The listing builds one solid part. Answer for the finished solid, in the listing's coordinates (mm). Face numbers are marked on the shaded views. A direction names the side the tool comes from. Round coordinates to 2 decimals unless told otherwise and drop trailing zeros. Write each loop counter-clockwise with the first axis right and the second up, starting at its lowest first coordinate (ties: lowest second). Pieces come first, ordered by that corner, then holes. Notation, with made-up numbers: M 15.5,19.25 L 56.5,19.25 A13 cw 56.5,40.25 Z; hole C -23.75,88.5 d3. An arc over 180 degrees is marked long. One line per item, written item: value. Start each with the question number.
(1) Section A-A (y = -11) is taken. Determine the outline of the cut face in (x, z), plus the area to 3 significant figures.
(2) Section C-C (y = -22) is taken. Determine the outline of the cut face in (x, z).
(3) Given P1, Ø0.7, axis at y = -26.5, z = 5, coming from the +X side; P2, Ø1.3, axis at x = 0, y = -22, coming from the -Z side; P3, Ø1, axis at y = -28, z = 4, coming from the +X side, each flat-ended and moving along its own axis, determine where each tip first touches the part or whether it passes through.
(4) For a pull along Y with two mould halves and no side action, classify the marked faces 1, 2, 3 and 4 as released by +Y, released by -Y, zero draft, split by the parting line, or undercut.
(5) For the marked faces 5, 6, 7 and 8, determine the directions among +Z, -Z, +X, -X, +Y, -Y from which every point of the face is accessible in a straight line to the end or side of a thin tool.
(6) Section B-B (x = 5) is taken. Determine the outline of the cut face in (y, z).
(7) Consider probe 1 along X at (y, z) = (-11, 1.55); probe 2 along X at (y, z) = (-12.5, 3); probe 3 along Y at (x, z) = (5, 2.8). Determine where each line is inside the solid, lowest interval first.
(8) Section D-D (z = 0.7) is taken. State how many separate pieces and enclosed holes the cut face has, plus the area to 3 significant figures.
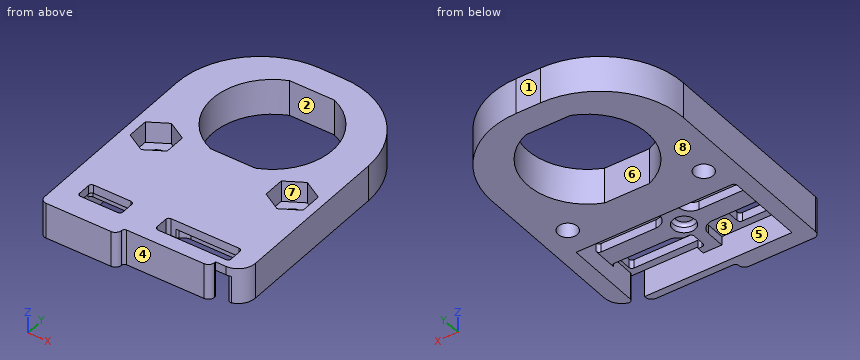
```python
from build123d import *

# Parameters (mm, degrees)
SKETCH_R        = 1.55
SKETCH_W        = 7
SKETCH_H        = 3
SKETCH_W_2      = 12
PAD_DEPTH       = 5.8
SKETCH005_W     = 25.7
SKETCH005_H     = 13
POCKET_DEPTH    = 3
SKETCH006_R     = 1.8
POCKET001_DEPTH = 1.4
POCKET002_DEPTH = 3.4
FILLET_R        = 1
FILLET001_R     = 0.5


with BuildPart() as part:
    # Sketch → Pad (new body)
    with BuildSketch(Plane.XY):
        with BuildLine():
            Line((-2, 13.5), (2, 13.5))
            ThreePointArc((15.5, 0), (11.545942, 9.545942), (2, 13.5))
            Line((15.5, 0), (15.5, -25.7))
            ThreePointArc((12.7, -28.5), (14.679899, -27.679899), (15.5, -25.7))
            Line((11, -28.5), (12.7, -28.5))
            Line((11, -29.7), (11, -28.5))
            Line((-3, -29.7), (11, -29.7))
            Line((-3, -31.15), (-3, -29.7))
            Line((-3, -31.15), (-15.5, -31.15))
            Line((-15.5, -31.15), (-15.5, 0))
            ThreePointArc((-2, 13.5), (-11.545942, 9.545942), (-15.5, 0))
        make_face()
        with Locations((-11, -11)):
            Circle(SKETCH_R, mode=Mode.SUBTRACT)
        with Locations((11, -11)):
            Circle(SKETCH_R, mode=Mode.SUBTRACT)
        with BuildLine():
            ThreePointArc((-3.618011, 9), (-9.7, 0), (-3.618011, -9))
            Line((3.618011, -9), (-3.618011, -9))
            ThreePointArc((3.618011, -9), (9.7, 0), (3.618011, 9))
            Line((-3.618011, 9), (3.618011, 9))
        make_face(mode=Mode.SUBTRACT)
        with Locations((-8.66, -25.81)):
            Rectangle(SKETCH_W, SKETCH_H, mode=Mode.SUBTRACT)
        with Locations((6.35, -25.81)):
            Rectangle(SKETCH_W_2, SKETCH_H, mode=Mode.SUBTRACT)
    extrude(amount=PAD_DEPTH)

    # Sketch005 (on Face26 of Pad) → Pocket (cut)
    with BuildSketch(Plane(origin=(0, 0, 0), x_dir=(1, 0, 0), z_dir=(0, 0, -1))):
        with Locations((0, 22)):
            Rectangle(SKETCH005_W, SKETCH005_H)
    extrude(amount=-POCKET_DEPTH, mode=Mode.SUBTRACT)

    # Sketch006 (on Face32 of Pocket) → Pocket001 (cut)
    with BuildSketch(Plane(origin=(0, 0, 3), x_dir=(1, 0, 0), z_dir=(0, 0, -1))):
        with Locations((0, 22)):
            Circle(SKETCH006_R)
        with BuildLine():
            Line((-12.85, 20.5), (-3.5, 20.5))
            ThreePointArc((-1.5, 18.5), (-2.085786, 19.914214), (-3.5, 20.5))
            Line((-1.5, 18.5), (-1.5, 15.5))
            Line((-1.5, 15.5), (-12.85, 15.5))
            Line((-12.85, 15.5), (-12.85, 20.5))
        make_face()
        with BuildLine():
            Line((1.5, 15.5), (12.85, 15.5))
            Line((12.85, 15.5), (12.85, 20.5))
            Line((12.85, 20.5), (3.5, 20.5))
            ThreePointArc((3.5, 20.5), (2.085786, 19.914214), (1.5, 18.5))
            Line((1.5, 18.5), (1.5, 15.5))
        make_face()
        with BuildLine():
            Line((-12.85, 23.5), (-3.5, 23.5))
            ThreePointArc((-3.5, 23.5), (-2.085786, 24.085786), (-1.5, 25.5))
            Line((-1.5, 25.5), (-1.5, 28.5))
            Line((-1.5, 28.5), (-12.85, 28.5))
            Line((-12.85, 28.5), (-12.85, 23.5))
        make_face()
        with BuildLine():
            Line((1.5, 28.5), (12.85, 28.5))
            Line((12.85, 28.5), (12.85, 23.5))
            Line((12.85, 23.5), (3.5, 23.5))
            ThreePointArc((1.5, 25.5), (2.085786, 24.085786), (3.5, 23.5))
            Line((1.5, 25.5), (1.5, 28.5))
        make_face()
    extrude(amount=-POCKET001_DEPTH, mode=Mode.SUBTRACT)

    # Sketch001 (on Face5 of Pocket001) → Pocket002 (cut)
    with BuildSketch(Plane.XY.offset(5.8)):
        Polygon((-8, -12.732051), (-8, -9.267949), (-11, -7.535898), (-14, -9.267949), (-14, -12.732051), (-11, -14.464102), align=None)
        Polygon((14, -12.732051), (14, -9.267949), (11, -7.535898), (8, -9.267949), (8, -12.732051), (11, -14.464102), align=None)
    extrude(amount=-POCKET002_DEPTH, mode=Mode.SUBTRACT)

    # Fillet
    fillet_edges = [part.edges().sort_by_distance(p)[0] for p in [
        (-15.5, -31.15, 2.9),
        (-3, -31.15, 2.9),
        (11, -29.7, 2.9),
    ]]
    fillet(fillet_edges, radius=FILLET_R)

    # Fillet001
    fillet001_edges = [part.edges().sort_by_distance(p)[0] for p in [
        (12.85, -23.5, 3.7),
        (12.85, -20.5, 3.7),
        (-12.85, -20.5, 3.7),
        (-12.85, -23.5, 3.7),
        (-1.8, -22, 4.4),
        (0.35, -27.31, 4.4),
        (0.35, -24.31, 4.4),
        (1.892549, -24.31, 3.7),
        (-3, -29.7, 2.9),
        (12.35, -27.31, 5.1),
        (12.35, -24.31, 5.1),
        (-5.16, -27.31, 5.1),
        (-5.16, -24.31, 5.1),
        (-12.16, -24.31, 5.1),
        (-12.16, -27.31, 5.1),
        (-12.85, -15.5, 1.5),
        (12.85, -28.495979, 1.5),
    ]]
    fillet(fillet001_edges, radius=FILLET001_R)


solid = part.part
```
Recorded:
1. outline: M -15.5,0 L -12.55,0 L -12.55,2.4 L -14,2.4 L -14,5.8 L -15.5,5.8 Z; M -9.45,0 L 9.45,0 L 9.45,2.4 L 8,2.4 L 8,5.8 L -8,5.8 L -8,2.4 L -9.45,2.4 Z; M 12.55,0 L 15.5,0 L 15.5,5.8 L 14,5.8 L 14,2.4 L 12.55,2.4 Z
1. area: 124 mm2
2. outline: M -15.5,0 L -12.85,0 L -12.85,3 L -1.8,3 L -1.8,3.9 A0.5 cw -1.3,4.4 L 1.3,4.4 A0.5 cw 1.8,3.9 L 1.8,3 L 12.85,3 L 12.85,0 L 15.5,0 L 15.5,5.8 L -15.5,5.8 Z
3. P1: stops at x = 15.46
3. P2: stops at z = 4.4
3. P3: stops at x = 14.84
4. face 1: released by +Y
4. face 2: undercut
4. face 3: undercut
4. face 4: released by -Y
5. face 5: -Z
5. face 6: +Z, -Z
5. face 7: +Z
5. face 8: -Z, +X, -X, +Y, -Y
6. outline: M -29.7,0 L -28.5,0 L -28.5,4.4 L -27.31,4.4 L -27.31,5.8 L -29.7,5.8 Z; M -24.31,4.4 L -23.5,4.4 L -23.5,3 L -20.5,3 L -20.5,4.4 L -15.5,4.4 L -15.5,0 L -8.31,0 L -8.31,5.8 L -24.31,5.8 Z; M 8.31,0 L 13.16,0 L 13.16,5.8 L 8.31,5.8 Z
7. probe 1: x = -15.5 to -12.55, -9.45 to 9.45, 12.55 to 15.5
7. probe 2: x = -15.5 to -14, -8 to 8, 14 to 15.5
7. probe 3: y = -29.7 to -28.5, -15.5 to -8.31, 8.31 to 13.16
8. separate pieces: 1
8. enclosed holes: 3
8. area: 633 mm2
